Input: part model. Units: mm. Frame: model coordinates. Give positions to 0.01 mm unless a question says otherwise; leave off trailing zeros. Order: outer loops, then holes, each group sorted by start corner. A loop starts at its lowest first (then second) coordinate and runs counter-clockwise, first axis right, second up. Notation, with made-up numbers: (76.25, 71) - (117.25, 71) arc R24 cw to (117.25, 102) - close; hole circle Ø3 at (37, 26). An arc over 180 degrees is marked (long way). Use a Markdown table: item, result.
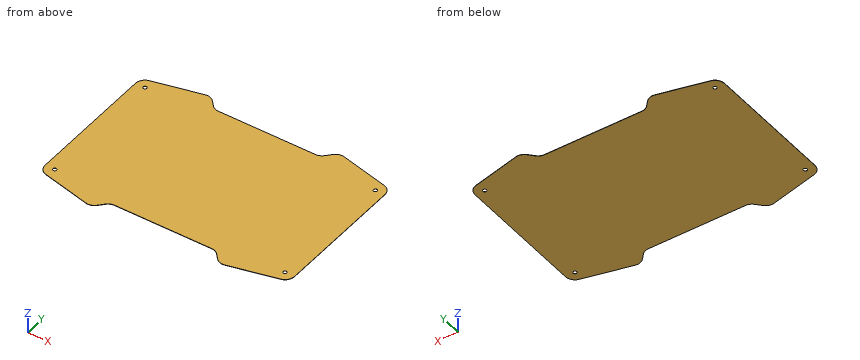
from build123d import *

# Parameters (mm, degrees)
F1_DEPTH = 0.37592
F2_R     = 12.7
F4_D     = 4.7625
F4_DEPTH = 6.731


with BuildPart() as f1:
    # F0 (on Top) → F1 (new body)
    with BuildSketch(Plane.XY):
        Polygon((165.1, -95.25), (165.1, 95.25), (84.778147, 114.3), (69.85, 97.876274), (0, 97.876274), (-69.85, 97.876274), (-84.778147, 114.3), (-165.1, 95.25), (-165.1, -95.25), (-84.778147, -114.3), (-69.85, -97.876274), (0, -97.876274), (69.85, -97.876274), (84.778147, -114.3), align=None)
    extrude(amount=F1_DEPTH)

    # F2
    f2_edges = [f1.edges().sort_by_distance(p)[0] for p in [
        (-165.1, -95.25, 0.18796),
        (-84.778147, -114.3, 0.18796),
        (-69.85, -97.876274, 0.18796),
        (69.85, -97.876274, 0.18796),
        (84.778147, -114.3, 0.18796),
        (165.1, -95.25, 0.18796),
        (165.1, 95.25, 0.18796),
        (84.778147, 114.3, 0.18796),
        (69.85, 97.876274, 0.18796),
        (-69.85, 97.876274, 0.18796),
        (-84.778147, 114.3, 0.18796),
        (-165.1, 95.25, 0.18796),
    ]]
    fillet(f2_edges, radius=F2_R)

    # F4
    with Locations(Plane.XY.offset(0.37592)):
        with Locations((152.4, -85.209768), (-152.4, -85.209768), (-152.4, 85.209768), (152.4, 85.209768)):
            Hole(F4_D / 2, depth=F4_DEPTH)


solid = f1.part
1. Material intervals for line 1 along Y through (x, z) = (35.5, 0.05); line 2 along Y through (x, z) = (152.4, 0.25); line 3 along X through (y, z) = (84, 0.1), sorted ascending.
Response:
| item | result |
|---|---|
| line 1 | y = -97.88 to 97.88 |
| line 2 | y = -98.26 to -87.59, -82.83 to 82.83, 87.59 to 98.26 |
| line 3 | x = -165.1 to -154.45, -150.35 to 150.35, 154.45 to 165.1 |
2. Section query C-C (x = -118.5). Return loops of the section in (y, z).
Response:
| item | result |
|---|---|
| outline | (-106.3, 0) - (106.3, 0) - (106.3, 0.38) - (-106.3, 0.38) - close |
3. Section query B-B (x = -46). Return loops of the section in (y, z), then the cut area to 3 significant figures.
Response:
| item | result |
|---|---|
| outline | (-97.88, 0) - (97.88, 0) - (97.88, 0.38) - (-97.88, 0.38) - close |
| area | 73.6 mm^2 |
4. Section query A-A (z = 0.2). Return loops of the section in (x, y), then the cut area to 3 significant figures.
Response:
| item | result |
|---|---|
| outline | (-165.1, -85.21) arc R12.7 ccw to (-155.33, -97.57) - (-92.07, -112.57) arc R12.7 ccw to (-79.74, -108.76) - (-73.63, -102.03) arc R12.7 cw to (-64.23, -97.88) - (64.23, -97.88) arc R12.7 cw to (73.63, -102.03) - (79.74, -108.76) arc R12.7 ccw to (92.07, -112.57) - (155.33, -97.57) arc R12.7 ccw to (165.1, -85.21) - (165.1, 85.21) arc R12.7 ccw to (155.33, 97.57) - (92.07, 112.57) arc R12.7 ccw to (79.74, 108.76) - (73.63, 102.03) arc R12.7 cw to (64.23, 97.88) - (-64.23, 97.88) arc R12.7 cw to (-73.63, 102.03) - (-79.74, 108.76) arc R12.7 ccw to (-92.07, 112.57) - (-155.33, 97.57) arc R12.7 ccw to (-165.1, 85.21) - close; hole circle Ø4.76 at (-152.4, -85.21); hole circle Ø4.76 at (-152.4, 85.21); hole circle Ø4.76 at (152.4, -85.21); hole circle Ø4.76 at (152.4, 85.21) |
| area | 67,200 mm^2 |
